```python
from build123d import *

# Parameters (mm, degrees)
SKETCH1_W                = 53
SKETCH1_H                = 15.35
SKETCH1_R                = 1.6
SKETCH1_R_2              = 2.6
BOSS_EXTRUDE1_DEPTH      = 10
BOSS_EXTRUDE2_DEPTH      = 4.325
BOSS_EXTRUDE2_DEPTH_BACK = 19.675
CUT_EXTRUDE1_DEPTH       = 20.675
CUT_EXTRUDE2_DEPTH       = 4
SKETCH5_R                = 2.6
BOSS_EXTRUDE3_DEPTH      = 0.4


with BuildPart() as part:
    # Sketch1 → Boss-Extrude1 (new body)
    with BuildSketch(Plane(origin=(0, 0, 0), x_dir=(1, 0, 0), z_dir=(0, 1, 0))):
        with Locations((46.893734614, 0)):
            Rectangle(SKETCH1_W, SKETCH1_H)
        with Locations((52.893734614, 0)):
            Circle(SKETCH1_R, mode=Mode.SUBTRACT)
        with Locations((24.893734614, 0)):
            Circle(SKETCH1_R, mode=Mode.SUBTRACT)
        with Locations((66.393734614, 0)):
            Circle(SKETCH1_R_2, mode=Mode.SUBTRACT)
    extrude(amount=BOSS_EXTRUDE1_DEPTH)

    # Sketch2 → Boss-Extrude2 (add, two sides)
    with BuildSketch(Plane(origin=(0, 0, -7.675), x_dir=(-1, 0, 0), z_dir=(0, 0, -1))) as boss_extrude2_sk:
        with BuildLine():
            Line((-44.801648562, 14.038617938), (-47.002272565, 16.170952878))
            ThreePointArc((-47.002272565, 16.170952878), (-48.777803829, 13.043328345), (-49.393734614, 9.5))
            Line((-49.393734614, 9.5), (-49.393734614, 0))
            Line((-49.393734614, 0), (-28.393734614, 0))
            Line((-28.393734614, 0), (-28.393734614, 9.5))
            ThreePointArc((-28.393734614, 9.5), (-29.451814157, 14.09348866), (-32.412808532, 17.761210391))
            Line((-32.412808532, 17.761210391), (-34.628407423, 15.608148979))
            ThreePointArc((-34.628407423, 15.608148979), (-37.757785789, 2.137111962), (-44.801648562, 14.038617938))
        make_face()
    extrude(amount=BOSS_EXTRUDE2_DEPTH)
    extrude(boss_extrude2_sk.sketch, amount=-BOSS_EXTRUDE2_DEPTH_BACK)

    # Sketch3 → Cut-Extrude1 (cut, through all)
    with BuildSketch(Plane.XY.offset(7.675)):
        with BuildLine():
            Line((46.326937154, 10), (31.460532075, 10))
            ThreePointArc((31.460532075, 10), (38.893734614, 2.05), (46.326937154, 10))
        make_face()
    extrude(amount=-CUT_EXTRUDE1_DEPTH, mode=Mode.SUBTRACT)

    # Sketch4 → Cut-Extrude2 (cut)
    with BuildSketch(Plane.XZ):
        Polygon((62.366716487, 2.325), (62.366716487, -2.325), (66.393734614, -4.65), (70.420752742, -2.325), (70.420752742, 2.325), (66.393734614, 4.65), align=None)
    extrude(amount=-CUT_EXTRUDE2_DEPTH, mode=Mode.SUBTRACT)

    # Sketch5 → Boss-Extrude3 (add)
    with BuildSketch(Plane.XZ.offset(-4)):
        with Locations((66.393734614, 0)):
            Circle(SKETCH5_R)
    extrude(amount=-BOSS_EXTRUDE3_DEPTH)


solid = part.part
```
Check sheet for the modelled part. Datum: model origin and axes. Units: mm. A direction names the side the tool comes from. Round coordinates to 2 decimals unless told otherwise and drop trailing zeros. Loops run counter-clockwise (first coordinate to the right, second up) from the corner with the lowest first, then second, coordinate; pieces in that order, holes last. Notation, with made-up numbers: (6, -26.5) -> (26, -26.5) arc R12 ccw to (26, -21.5) -> close; hole circle Ø11 at (89.5, 5.25). An arc over 180 degrees is marked (long way). Answer in a Markdown table with one row per item.
Q1. Sectioned sample at A-A on z = 0. Enter the section's corners in (x, y).
Data:
| item | result |
|---|---|
| outline | (20.39, 0) -> (23.29, 0) -> (23.29, 10) -> (20.39, 10) -> close; (26.49, 0) -> (51.29, 0) -> (51.29, 10) -> (49.38, 10) arc R10.5 ccw to (47, 16.17) -> (44.8, 14.04) arc R7.45 cw (long way) to (34.63, 15.61) -> (32.41, 17.76) arc R10.5 ccw to (28.41, 10) -> (26.49, 10) -> close; (54.49, 0) -> (62.37, 0) -> (62.37, 4) -> (70.42, 4) -> (70.42, 0) -> (73.39, 0) -> (73.39, 10) -> (68.99, 10) -> (68.99, 4.4) -> (63.79, 4.4) -> (63.79, 10) -> (54.49, 10) -> close |
Q2. Sectioned sample at B-B on y = 7.5. Enter the section's corners in (x, z) (3 decimals), then the cut area to 3 significant figures.
Data:
| item | result |
|---|---|
| outline | (20.394, -7.675) -> (28.394, -7.675) -> (28.394, -12) -> (31.717, -12) -> (31.717, 12) -> (28.394, 12) -> (28.394, 7.675) -> (20.394, 7.675) -> close; (46.07, -12) -> (49.394, -12) -> (49.394, -7.675) -> (73.394, -7.675) -> (73.394, 7.675) -> (49.394, 7.675) -> (49.394, 12) -> (46.07, 12) -> close; hole circle Ø3.2 at (24.894, 0); hole circle Ø3.2 at (52.894, 0); hole circle Ø5.2 at (66.394, 0) |
| area | 613 mm^2 |
Q3. Thickness scan on L1, parallel to X at y = 7.8, z = 0; L2, parallel to X at y = 4.25, z = 0; L3, parallel to X at y = 9.5, z = 4. Record the ranges inside material, lowest first.
Data:
| item | result |
|---|---|
| L1 | x = 20.39 to 23.29, 26.49 to 31.64, 46.15 to 51.29, 54.49 to 63.79, 68.99 to 73.39 |
| L2 | x = 20.39 to 23.29, 26.49 to 33.61, 44.18 to 51.29, 54.49 to 73.39 |
| L3 | x = 20.39 to 31.44, 46.34 to 73.39 |
Q4. Release check for a two-part mould opening along X. For faces 1 (the face through (39, 1, 12)), 2 (the face through (33.505, 16.7, -0.168)), 3 (the face through (28.394, 5, 10)), 4 (the face through (73.394, 5, 0)) record: released by +X, released by -X, zero draft, split by the parting line, or undercut.
Data:
| item | result |
|---|---|
| face 1 | zero draft |
| face 2 | undercut |
| face 3 | released by -X |
| face 4 | released by +X |
Q5. Set-up check for faces 5 (the face through (24, 5, 7.675)), 6 (the face through (49.394, 5, -10)), 7 (the face through (66, 4, 0)): record each of +Z, -Z, +X, -X, +Y, -Y from which the full face is reachable in a straight line by a thin tool's end or side.
Data:
| item | result |
|---|---|
| face 5 | +Z, -X, +Y, -Y |
| face 6 | -Z, +X, +Y, -Y |
| face 7 | -Y |
Q6. Sectioned sample at C-C on z = 9.75. Enter the section's corners in (x, y).
Data:
| item | result |
|---|---|
| outline | (28.39, 0) -> (49.39, 0) -> (49.39, 9.5) arc R10.5 ccw to (47, 16.17) -> (44.8, 14.04) arc R7.45 cw (long way) to (34.63, 15.61) -> (32.41, 17.76) arc R10.5 ccw to (28.39, 9.5) -> close |
Q7. Go/stop test with flat-tipped pins: P1, Ø12.5, axis at x = 60, z = 2.5, coming from the +Y side; P2, Ø3.5, axis at y = 4, z = -9.5, coming from the -X side; P3, Ø2.5, axis at x = 65.5, z = 2, coming from the -Y side. Record where each tip stops, or that it passes through.
Data:
| item | result |
|---|---|
| P1 | stops at y = 10 |
| P2 | stops at x = 28.39 |
| P3 | stops at y = 4 |
Q8. Sectioned sample at D-D on y = 13.5. Enter the section's corners in (x, z).
Data:
| item | result |
|---|---|
| outline | (29.19, -12) -> (32.61, -12) -> (32.61, 12) -> (29.19, 12) -> close; (45.18, -12) -> (48.6, -12) -> (48.6, 12) -> (45.18, 12) -> close |
